Autodesk Inventor part; units mm, degrees
ref_plane "YZ Plane" through (0, 0, 0) normal (1, 0, 0) x (0, 1, 0)
ref_plane "XZ Plane" through (0, 0, 0) normal (0, 1, 0) x (-1, 0, 0)
ref_plane "XY Plane" through (0, 0, 0) normal (0, 0, 1) x (1, 0, 0)
sketch "Sketch1" plane through (0, 0, 0) normal (0, 1, 0) x (-1, 0, 0)
  circle A0 centre (0, 0) radius 12.7
  dimension "d0" = 25.4
extrude "Extrusion1" add sketch "Sketch1" along normal blind 65.8812
fillet "Fillet1" radius 1.27 2 edges at (12.7, 65.8812, 0) (12.7, 0, 0)
sketch "Sketch2" plane through (0, 65.8812, 0) normal (0, 1, 0) x (1, 0, 0)
  circle A0 centre (0, 0) radius 9.1995
  arc A1 (-8.3949, -3.7625) -> (-8.3949, 3.7625) centre (-7.9295, 0) ccw
  arc A2 (3.7625, -8.3949) -> (-3.7625, -8.3949) centre (0, -7.9295) ccw
  arc A3 (8.3949, 3.7625) -> (8.3949, -3.7625) centre (7.9295, 0) ccw
  arc A4 (-3.7625, 8.3949) -> (3.7625, 8.3949) centre (0, 7.9295) ccw
  circle A5 centre (0, 0) radius 7.9295 construction
  line L0 (-3.7625, -8.3949) -> (3.7625, -8.3949) construction
  line L1 (8.3949, -3.7625) -> (8.3949, 3.7625) construction
  line L2 (3.7625, 8.3949) -> (-3.7625, 8.3949) construction
  line L3 (-8.3949, 3.7625) -> (-8.3949, -3.7625) construction
  point P0 (3.7625, 8.3949)
  point P1 (-3.7625, 8.3949)
  point P2 (-3.7625, -8.3949)
  point P3 (3.7625, -8.3949)
  point P4 (8.3949, -3.7625)
  point P5 (8.3949, 3.7625)
  dimension "d6" = 360
  dimension "d8" = 1.27
extrude "Extrusion2" add sketch "Sketch2" along normal blind 2 contours A3 A0 A2 A1 A4
fillet "Fillet2" radius 2.54 4 edges at (6.5051, 67.8812, 6.5051) (-6.5051, 67.8812, 6.5051) (-6.5051, 67.8812, -6.5051) (6.5051, 67.8812, -6.5051)
properties part number "BigBattery"
Input: part model. Units: mm. Frame: model coordinates. A direction names the side the tool comes from. Round coordinates to 2 decimals unless told otherwise and drop trailing zeros. Write each loop counter-clockwise with the first axis right and the second up, starting at its lowest first coordinate (ties: lowest second). Pieces come first, ordered by that corner, then holes. Notation, with made-up numbers: (3, 77.25) - (16, 77.25) arc R18 ccw to (16, 93.25) - close; hole circle Ø1 at (63.25, -40). An arc over 180 degrees is marked (long way). Write item = value, one per line.
(1) Access query for faces 4 (the flat face through (0, 0, 0)), 5 (the flat face through (-5, 65.881, 0)). Directions: +Z, -Z, +X, -X, +Y, -Y. A direction counts if a zero-diameter tool reaches every point of the face in a straight line with its end or side. Return the directions, or none.
Geometry check:
face_4 = +Z, -Z, +X, -X, -Y
face_5 = +Y
(2) Section query C-C on y = 58.5. Output: boundary loops of the cut face in (x, z), then the cut area to 3 significant figures.
Geometry check:
outline = circle Ø25.4 at (0, 0)
area = 507 mm^2
(3) Pull-direction query (Z, two-part tool) for faces 1 (the cylindrical face through (2.75, 32.5, 12.4)), 2 (the flat face through (0, 67.881, 0)), 3 (the cylindrical face through (-4.14, 66.87, -0.09)); classes: +Z half, -Z half, draft (parallel to the pull), parting line (faces both ways), or undercut.
Geometry check:
face_1 = parting line
face_2 = draft
face_3 = undercut
(4) Section query A-A on x = 0. Output: boundary loops of the cut face in (y, z).
Geometry check:
outline = (0, -11.43) arc R1.27 ccw to (1.27, -12.7) - (64.61, -12.7) arc R1.27 ccw to (65.88, -11.43) - (65.88, -4.14) - (67.88, -4.14) - (67.88, 4.14) - (65.88, 4.14) - (65.88, 11.43) arc R1.27 ccw to (64.61, 12.7) - (1.27, 12.7) arc R1.27 ccw to (0, 11.43) - close
(5) Material intervals for probe 1 along Y at (x, z) = (6.25, -8.75); probe 2 along Z at (x, y) = (-11.25, 41); probe 3 along Z at (x, y) = (0, 67.25), sorted ascending.
Geometry check:
probe_1 = 0 to 65.88
probe_2 = -5.89 to 5.89
probe_3 = -4.14 to 4.14
(6) Contact query for flat-ended pins moving along their axis: pin 1 Ø8 at (x, y) = (9.5, 43.5) entering from +Z; pin 2 Ø1.5 at (x, y) = (5.5, 43) entering from +Z; pin 3 Ø8 at (y, z) = (12.5, -9) entering from -X. Output: stop coordinate, or through.
Geometry check:
pin_1 = 11.45
pin_2 = 11.78
pin_3 = -11.67
(7) Section query B-B on z = 0. Output: boundary loops of the cut face in (x, y), then the cut area to 3 significant figures.
Geometry check:
outline = (-12.7, 1.27) arc R1.27 ccw to (-11.43, 0) - (11.43, 0) arc R1.27 ccw to (12.7, 1.27) - (12.7, 64.61) arc R1.27 ccw to (11.43, 65.88) - (4.14, 65.88) - (4.14, 67.88) - (-4.14, 67.88) - (-4.14, 65.88) - (-11.43, 65.88) arc R1.27 ccw to (-12.7, 64.61) - close
area = 1,690 mm^2
